from build123d import *

# Parameters (mm, degrees)
EXTRUDE_1_DEPTH   = 14
SKETCH_1_R        = 6.5
EXTRUDE_1_2_DEPTH = 14
EXTRUDE_1_3_DEPTH = 14
SKETCH_2_W        = 39
SKETCH_2_H        = 13
EXTRUDE_2_DEPTH   = 6
SKETCH_3_R        = 6.5
EXTRUDE_3_DEPTH   = 14
SKETCH_4_W        = 39
SKETCH_4_H        = 13
EXTRUDE_4_DEPTH   = 6
SKETCH_5_W        = 45
SKETCH_5_H        = 26
EXTRUDE_5_DEPTH   = 8


with BuildPart() as part:
    # Sketch 1 → Extrude 1 (new body)
    with BuildSketch(Plane(origin=(0, 0, 0), x_dir=(1, 0, 0), z_dir=(0, 1, 0))):
        with BuildLine():
            Line((0, 13), (0, 0))
            Line((0, 0), (6.538518603, 0))
            ThreePointArc((6.538518603, 0), (5, 6.5), (6.538518603, 13))
            Line((6.538518603, 13), (0, 13))
        make_face()
    extrude(amount=EXTRUDE_1_DEPTH)



with BuildPart() as body_2:
    # Sketch 1 → Extrude 1 2 (new body)
    with BuildSketch(Plane(origin=(0, 0, 0), x_dir=(1, 0, 0), z_dir=(0, 1, 0))):
        with Locations(Location((19.5, 6.5, 0), (0, 0, 270))):
            Circle(SKETCH_1_R)
    extrude(amount=EXTRUDE_1_2_DEPTH)


with BuildPart() as body_3:
    # Sketch 1 → Extrude 1 3 (new body)
    with BuildSketch(Plane(origin=(0, 0, 0), x_dir=(1, 0, 0), z_dir=(0, 1, 0))):
        with BuildLine():
            ThreePointArc((34, 6.5), (33.61012899, 3.160200624), (32.461481397, 0))
            Line((32.461481397, 0), (39, 0))
            Line((39, 0), (39, 13))
            Line((39, 13), (32.461481397, 13))
            ThreePointArc((32.461481397, 13), (33.61012899, 9.839799376), (34, 6.5))
        make_face()
    extrude(amount=EXTRUDE_1_3_DEPTH)


with BuildPart() as part_1:
    add(part.part)

    add(body_2.part)  # Extrude 2 merges body 2

    add(body_3.part)  # Extrude 2 merges body 3
    # Sketch 2 → Extrude 2 (add)
    with BuildSketch(Plane.XZ):
        with Locations((19.5, -6.5)):
            Rectangle(SKETCH_2_W, SKETCH_2_H)
    extrude(amount=EXTRUDE_2_DEPTH)

    # Sketch 3 → Extrude 3 (add)
    with BuildSketch(Plane(origin=(0, 14, 0), x_dir=(1, 0, 0), z_dir=(0, 1, 0))):
        with Locations(Location((19.5, 6.5, 0), (0, 0, 270))):
            Circle(SKETCH_3_R)
        with BuildLine():
            Line((32.461481397, 0), (39, 0))
            Line((39, 0), (39, 13))
            Line((39, 13), (32.461481397, 13))
            ThreePointArc((32.461481397, 13), (34, 6.5), (32.461481397, 0))
        make_face()
        with BuildLine():
            Line((6.538518603, 13), (0, 13))
            Line((0, 13), (0, 0))
            Line((0, 0), (6.538518603, 0))
            ThreePointArc((6.538518603, 0), (5, 6.5), (6.538518603, 13))
        make_face()
    extrude(amount=EXTRUDE_3_DEPTH)

    # Sketch 4 → Extrude 4 (add)
    with BuildSketch(Plane(origin=(0, 28, 0), x_dir=(1, 0, 0), z_dir=(0, 1, 0))):
        with Locations((19.5, 6.5)):
            Rectangle(SKETCH_4_W, SKETCH_4_H)
    extrude(amount=EXTRUDE_4_DEPTH)

    # Sketch 5 → Extrude 5 (add)
    with BuildSketch(Plane(origin=(0, 34, 0), x_dir=(1, 0, 0), z_dir=(0, 1, 0))):
        with Locations((19.5, 6.5)):
            Rectangle(SKETCH_5_W, SKETCH_5_H)
    extrude(amount=EXTRUDE_5_DEPTH)


solid = part_1.part
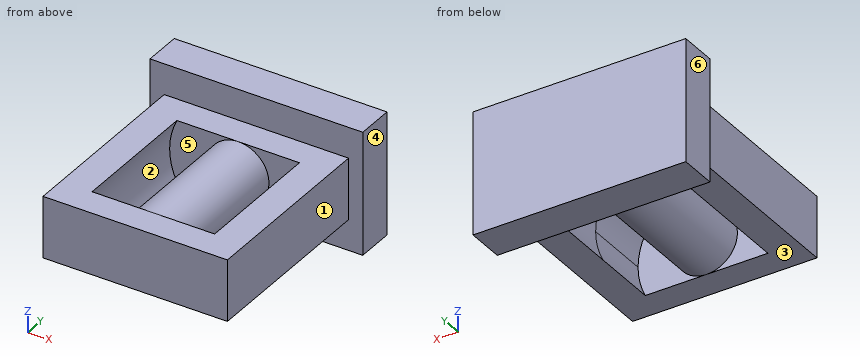
Read the model definition and answer for the solid it produces. Units are mm, in the model's axes. Face numbers are marked on the shaded views. A direction names the side the tool comes from. Round coordinates to 2 decimals unless told otherwise and drop trailing zeros. Write each loop counter-clockwise with the first axis right and the second up, starting at its lowest first coordinate (ties: lowest second). Pieces come first, ordered by that corner, then holes. Notation, with made-up numbers: (13, 18) - (26, 18) arc R28 cw to (26, 48) - close; hole circle Ø7 at (73, 4). An arc over 180 degrees is marked (long way). Use a Markdown table: item, result.
(1) The part is cut by section B-B (y = 3). Write down the section's boundary in (x, z).
Reported:
| item | result |
|---|---|
| outline | (0, -13) - (6.54, -13) arc R14.5 cw to (6.54, 0) - (0, 0) - close; circle Ø13 at (19.5, -6.5); (32.46, -13) - (39, -13) - (39, 0) - (32.46, 0) arc R14.5 cw to start |
(2) Straight lines are drawn through the part: line 1 along Y through (x, z) = (16, -0.25); line 2 along X through (y, z) = (19, -1.25); line 3 along Y through (x, z) = (25.5, 3). For each, find the intervals that lie inside material, in ascending order. Write a range as [from, to].
Reported:
| item | result |
|---|---|
| line 1 | [-6, 0], [28, 42] |
| line 2 | [0, 5.98], [15.67, 23.33], [33.02, 39] |
| line 3 | [34, 42] |
(3) The mould has two halves that part along X. Classify the marked faces 4, 5 and 6: released by +X, released by -X, zero draft, split by the parting line, or undercut.
Reported:
| item | result |
|---|---|
| face 4 | released by +X |
| face 5 | undercut |
| face 6 | released by -X |
(4) Each of these flat-tipped pins is pushed along its axis until it touches: pin 1 Ø6 at (y, z) = (10.5, -15) entering from -X; pin 2 Ø19.5 at (x, y) = (12, 21.5) entering from +Z; pin 3 Ø1.5 at (y, z) = (1.5, -4) entering from +X. Where does it stop, or does it pass through?
Reported:
| item | result |
|---|---|
| pin 1 | x = 0 |
| pin 2 | z = 0 |
| pin 3 | x = 39 |
(5) The part is cut by section C-C (x = 22). Write down the section's boundary in (y, z).
Reported:
| item | result |
|---|---|
| outline | (-6, -13) - (0, -13) - (0, -12.5) - (28, -12.5) - (28, -13) - (34, -13) - (34, -19.5) - (42, -19.5) - (42, 6.5) - (34, 6.5) - (34, 0) - (28, 0) - (28, -0.5) - (0, -0.5) - (0, 0) - (-6, 0) - close |
(6) Which of the six approach directions +Z, -Z, +X, -X, +Y, -Y give full straight-line access (tool end or side, diameter ignored) to the marked faces 1, 2 and 3?
Reported:
| item | result |
|---|---|
| face 1 | +Z, -Z, +X, -Y |
| face 2 | none |
| face 3 | -Z, +X, -X, -Y |
(7) The part is cut by section A-A (x = 7.5). Write down the section's boundary in (y, z).
Reported:
| item | result |
|---|---|
| outline | (-6, -13) - (0, -13) - (0, 0) - (-6, 0) - close; (28, -13) - (34, -13) - (34, -19.5) - (42, -19.5) - (42, 6.5) - (34, 6.5) - (34, 0) - (28, 0) - close |
(8) The part is cut by section D-D (z = -11.5). Write down the section's boundary in (x, y), then the cut area to 3 significant figures.
Reported:
| item | result |
|---|---|
| outline | (-3, 34) - (0, 34) - (0, -6) - (39, -6) - (39, 34) - (42, 34) - (42, 42) - (-3, 42) - close; hole (5.89, 0) - (15.35, 0) - (15.35, 28) - (5.89, 28) - close; hole (23.65, 0) - (33.11, 0) - (33.11, 28) - (23.65, 28) - close |
| area | 1,390 mm2 |
